Here's the drawing with two shaded views (mm, measured from the low corner). I have some questions. Round coordinates to 2 decimals unless told otherwise and drop trailing zeros. Loops run counter-clockwise (first coordinate to the right, second up) from the corner with the lowest first, then second, coordinate; pieces in that order, holes last. Notation, with made-up numbers: (10, 22) -> (35, 22) arc R24 ccw to (35, 39) -> close; hole circle Ø1 at (77, 67). An arc over 180 degrees is marked (long way). One line per item, written item: value. Start each with the question number.
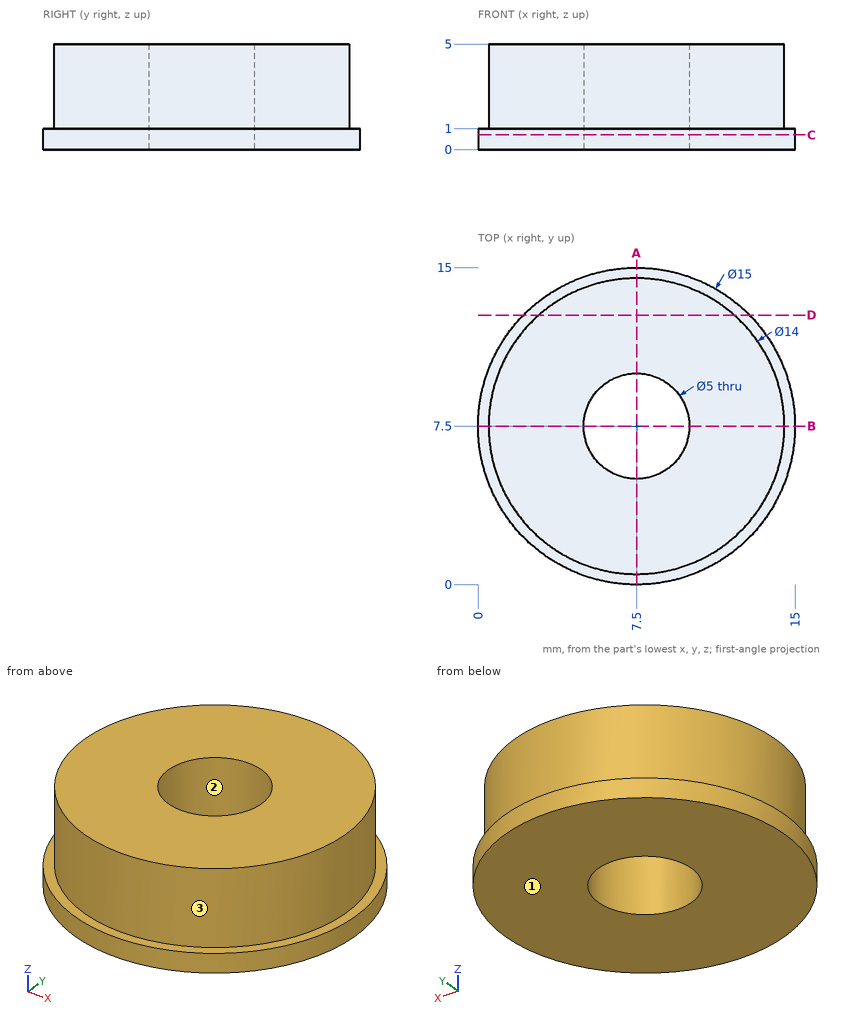
Q1. If we mould it in two halves opening along Y, with no side actions, what happens to the marked faces 1, 2 and 3? For each: released by +Y, released by -Y, zero draft, split by the parting line, or undercut.
Q2. Will these pins go through, and if not, where does the flat tip stop? P1, Ø2, axis at x = 9.5, z = 1.5, coming from the +Y side; P2, Ø4.5, axis at x = 5.5, y = 8.5, coming from the +Z side; P3, Ø1, axis at x = 5.5, z = 1, coming from the +Y side; P4, Ø1.5, axis at x = 10.5, z = 3.5, coming from the +Y side.
Q3. I want a section at D-D on y = 12.75. Please give me the cut outline in (x, z), plus the area to 3 significant figures.
Q4. If I drill on line 1 along Y through (x, z) = (7.5, 2.2); line 2 along Y through (x, z) = (5.5, 4.3); line 3 along Z through (x, y) = (14.25, 4.5), over which ranges is the centre line in solid material (lowest first)?
Q5. I want a section at A-A on x = 7.5. Please give me the cut outline in (y, z), plus the area to 3 significant figures.
Q6. I want a section at C-C on z = 0.7. Please give me the cut outline in (x, y), plus the area to 3 significant figures.
Answers below:
1. face 1: zero draft
1. face 2: undercut
1. face 3: split by the parting line
2. P1: stops at y = 14.91
2. P2: stops at z = 5
2. P3: stops at y = 14.85
2. P4: stops at y = 14.13
3. outline: (2.14, 0) -> (12.86, 0) -> (12.86, 1) -> (12.13, 1) -> (12.13, 5) -> (2.87, 5) -> (2.87, 1) -> (2.14, 1) -> close
3. area: 47.8 mm^2
4. line 1: y = 0.5 to 5, 10 to 14.5
4. line 2: y = 0.79 to 6, 9 to 14.21
4. line 3: z = 0 to 1
5. outline: (0, 0) -> (5, 0) -> (5, 5) -> (0.5, 5) -> (0.5, 1) -> (0, 1) -> close; (10, 0) -> (15, 0) -> (15, 1) -> (14.5, 1) -> (14.5, 5) -> (10, 5) -> close
5. area: 46.0 mm^2
6. outline: circle Ø15 at (7.5, 7.5); hole circle Ø5 at (7.5, 7.5)
6. area: 157 mm^2
